Could you check a few things on this model? Use its own coordinates, in mm. Face numbers are marked on the shaded views. Round coordinates to 2 decimals unless told otherwise and drop trailing zeros. Write each loop counter-clockwise with the first axis right and the second up, starting at its lowest first coordinate (ties: lowest second). Pieces come first, ordered by that corner, then holes. Notation, with made-up numbers: (-27.75, -21) -> (-11.75, -21) arc R27 ccw to (-11.75, -4) -> close; hole circle Ø9 at (-4, 87). An arc over 180 degrees is marked (long way). Return JSON: item names as keys, results as strings.
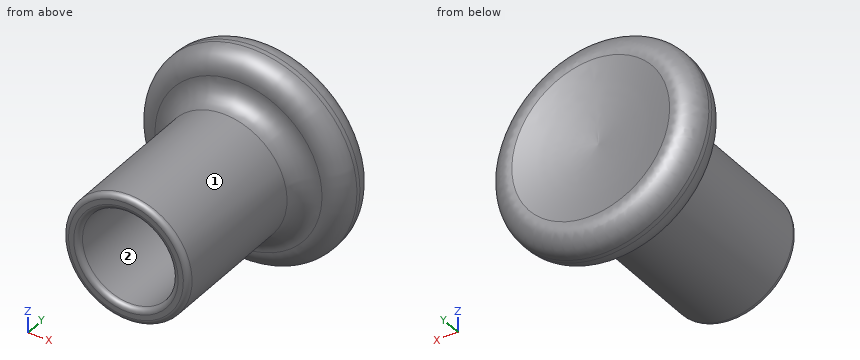
from build123d import *

# Parameters (mm, degrees)
SKETCH_1_R      = 6
SKETCH_1_R_2    = 4.5
EXTRUDE_1_DEPTH = 16
SKETCH_2_R      = 10
EXTRUDE_2_DEPTH = 5
FILLET_1_R      = 2
FILLET_2_R      = 0.5


with BuildPart() as part:
    # 草圖1 → 填料-伸長1 (new body)
    with BuildSketch(Plane(origin=(0, 0, 0), x_dir=(1, 0, 0), z_dir=(0, 1, 0))):
        with Locations(Location((0, 0, 0), (0, 0, 270))):
            Circle(SKETCH_1_R)
        with Locations(Location((0, 0, 0), (0, 0, 270))):
            Circle(SKETCH_1_R_2, mode=Mode.SUBTRACT)
    extrude(amount=EXTRUDE_1_DEPTH)

    # 草圖2 → 填料-伸長2 (add)
    with BuildSketch(Plane(origin=(0, 16, 0), x_dir=(1, 0, 0), z_dir=(0, 1, 0))):
        with Locations(Location((0, 0, 0), (0, 0, 270))):
            Circle(SKETCH_2_R)
    extrude(amount=EXTRUDE_2_DEPTH)

    # 草圖3 → 除料-旋轉1 (revolve, cut)
    with BuildSketch(Plane(origin=(0, 0, 0), x_dir=(0, 0, -1), z_dir=(1, 0, 0))):
        with BuildLine():
            Line((0, 21), (0, 19.316289144))
            add(Edge.make_bspline(
                [(-10, 21), (-5.090329438, 19.596139372), (0, 19.316289144)],
                knots=[0, 0, 0, 1, 1, 1], degree=2))
            Line((-10, 21), (0, 21))
        make_face()
    revolve(axis=Axis((0, 21, 0), (0, -1, 0)), mode=Mode.SUBTRACT)

    # 圓角1
    fillet_1_edges = [part.edges().sort_by_distance(p)[0] for p in [
        (0, 21, -10),
        (0, 16, -6),
        (0, 16, -10),
    ]]
    fillet(fillet_1_edges, radius=FILLET_1_R - 0.0001)  # a hair under: the kernel refuses the full size

    # 圓角2
    fillet_2_edges = [part.edges().sort_by_distance(p)[0] for p in [
        (0, 0, -6),
        (0, 0, -4.5),
    ]]
    fillet(fillet_2_edges, radius=FILLET_2_R)


solid = part.part
1) If I drill on probe 1 along X at (y, z) = (4.5, 0); probe 2 along Y at (x, z) = (-7.75, -2.5); probe 3 along Z at (x, y) = (2.5, 3.5), over which ranges is the centre line in solid material (lowest first)? Write a range as [from, to].
Return value:
{"probe 1": "[-6, -4.5], [4.5, 6]", "probe 2": "[16.01, 20.42]", "probe 3": "[-5.45, -3.74], [3.74, 5.45]"}
2) I want a section at A-A, the plane y = 13.5. Please give me the cut outline in (x, z), and give its area (3 significant figures).
Return value:
{"outline": "circle Ø12 at (0, 0); hole circle Ø9 at (0, 0)", "area": "49.5 mm²"}
3) Will these pins go through, and if not, where does the flat tip stop? pin 1 Ø5 at (y, z) = (7, -2) entering from -X; pin 2 Ø8 at (x, z) = (0, 0) entering from +Y; pin 3 Ø3 at (x, y) = (5.5, 5) entering from +Z; pin 4 Ø1.5 at (y, z) = (5.5, 7.5) entering from -X.
Return value:
{"pin 1": "x = -6", "pin 2": "y = 19.71", "pin 3": "z = 4.47", "pin 4": "through"}
4) Thinking about a two-plate mould opening in Z: for the marked faces 1 and 2, which applies, pulls with the +Z half, pulls with the -Z half, needs draft (parallel to the pull), parting line crosses it, or undercut?
Return value:
{"face 1": "parting line crosses it", "face 2": "undercut"}
